Here's how the part is built. I have some questions about the finished solid (model axes, mm). A direction names the side the tool comes from. Round coordinates to 2 decimals unless told otherwise and drop trailing zeros. Order: outer loops, then holes, each group sorted by start corner. A loop starts at its lowest first (then second) coordinate and runs counter-clockwise, first axis right, second up. Notation, with made-up numbers: M 80,-39 L 120,-39 A28 cw 120,-18 Z; hole C -13.75,73.5 d6. An arc over 180 degrees is marked long. Write each question's results on one line, items separated by ' | '. Start each with the question number.
```python
from build123d import *

# Parameters (mm, degrees)
SKETCH1_W           = 15.000000596
SKETCH1_H           = 15.000000597
BOSS_EXTRUDE1_DEPTH = 12.000000104
SKETCH2_W           = 8.999999613
SKETCH2_H           = 9.000003338
CUT_EXTRUDE1_DEPTH  = 11.002000072
SKETCH3_W           = 6.504997611
SKETCH3_H           = 6.504997611
CUT_EXTRUDE2_DEPTH  = 102.11874099
SKETCH4_W           = 3.00199911
SKETCH4_H           = 7.001999765
CUT_EXTRUDE3_DEPTH  = 1.501999795
SKETCH5_W           = 7.001999765
SKETCH5_H           = 3.002002835
CUT_EXTRUDE4_DEPTH  = 1.501999795
SKETCH6_W           = 7.001999765
SKETCH6_H           = 3.002002835
CUT_EXTRUDE5_DEPTH  = 1.502998173
SKETCH7_W           = 3.00199911
SKETCH7_H           = 7.001999765
CUT_EXTRUDE6_DEPTH  = 1.502998173
SKETCH9_W           = 2
SKETCH9_H           = 5.000000597
BOSS_EXTRUDE2_DEPTH = 5
SKETCH10_W          = 2
SKETCH10_H          = 5.000000597
BOSS_EXTRUDE3_DEPTH = 5
SKETCH11_R          = 1.6
CUT_EXTRUDE7_DEPTH  = 5


with BuildPart() as part:
    # Sketch1 → Boss-Extrude1 (new body)
    with BuildSketch(Plane(origin=(0, 0, 0), x_dir=(-1, 0, 0), z_dir=(0, 0, -1))):
        with Locations((47.499999404, 76.49999857)):
            Rectangle(SKETCH1_W, SKETCH1_H)
    extrude(amount=-BOSS_EXTRUDE1_DEPTH)

    # Sketch2 → Cut-Extrude1 (cut)
    with BuildSketch(Plane.XY.offset(12.000000104)):
        with Locations((-47.500001266, 76.375000179)):
            Rectangle(SKETCH2_W, SKETCH2_H)
    extrude(amount=-CUT_EXTRUDE1_DEPTH, mode=Mode.SUBTRACT)

    # Sketch3 → Cut-Extrude2 (cut, through all)
    with BuildSketch(Plane(origin=(0, 0, 0), x_dir=(-1, 0, 0), z_dir=(0, 0, -1))):
        with Locations((47.500498593, 76.375499367)):
            Rectangle(SKETCH3_W, SKETCH3_H)
    extrude(amount=-CUT_EXTRUDE2_DEPTH, mode=Mode.SUBTRACT)

    # Sketch4 → Cut-Extrude3 (cut)
    with BuildSketch(Plane(origin=(0, 71.87499851, 0), x_dir=(-1, 0, 0), z_dir=(0, 1, 0))):
        with Locations((47.500001267, 8.499000222)):
            Rectangle(SKETCH4_W, SKETCH4_H)
    extrude(amount=-CUT_EXTRUDE3_DEPTH, mode=Mode.SUBTRACT)

    # Sketch5 → Cut-Extrude4 (cut)
    with BuildSketch(Plane.ZY.offset(43.00000146)):
        with Locations((8.499000222, 76.375000179)):
            Rectangle(SKETCH5_W, SKETCH5_H)
    extrude(amount=-CUT_EXTRUDE4_DEPTH, mode=Mode.SUBTRACT)

    # Sketch6 → Cut-Extrude5 (cut)
    with BuildSketch(Plane(origin=(-52.000001073, 0, 0), x_dir=(0, 0, -1), z_dir=(1, 0, 0))):
        with Locations((-8.499000222, 76.375000179)):
            Rectangle(SKETCH6_W, SKETCH6_H)
    extrude(amount=-CUT_EXTRUDE5_DEPTH, mode=Mode.SUBTRACT)

    # Sketch7 → Cut-Extrude6 (cut)
    with BuildSketch(Plane.XZ.offset(-80.875001848)):
        with Locations((-47.500001267, 8.499000222)):
            Rectangle(SKETCH7_W, SKETCH7_H)
    extrude(amount=-CUT_EXTRUDE6_DEPTH, mode=Mode.SUBTRACT)

    # Sketch9 → Boss-Extrude2 (add)
    with BuildSketch(Plane.ZY.offset(54.999999702)):
        with Locations((1, 76.49999857)):
            Rectangle(SKETCH9_W, SKETCH9_H)
    extrude(amount=BOSS_EXTRUDE2_DEPTH)

    # Sketch10 → Boss-Extrude3 (add)
    with BuildSketch(Plane(origin=(-39.999999106, 0, 0), x_dir=(0, 0, -1), z_dir=(1, 0, 0))):
        with Locations((-1, 76.49999857)):
            Rectangle(SKETCH10_W, SKETCH10_H)
    extrude(amount=BOSS_EXTRUDE3_DEPTH)

    # Sketch11 → Cut-Extrude7 (cut)
    with BuildSketch(Plane.XY.offset(2)):
        with Locations((-37.499999106, 76.499998569)):
            Circle(SKETCH11_R)
        with Locations((-57.499999702, 76.499998569)):
            Circle(SKETCH11_R)
    extrude(amount=-CUT_EXTRUDE7_DEPTH, mode=Mode.SUBTRACT)


solid = part.part
```
(1) I want a section at B-B on z = 7.75. Write out the boundary of the cut face in (x, y) (3 decimals).
(2) I want a section at A-A on x = -37.5. Write out the boundary of the cut face in (y, z), and give its area (3 significant figures).
(3) If we mould it in two halves opening along Y, with no side actions, what happens to faces 4 (the flat face through (-47, 80, 0)), 5 (the flat face through (-48, 82.378, 9)), 6 (the flat face through (-38, 79, 1))? For each: pulls with the +Y half, pulls with the -Y half, needs draft (parallel to the pull), parting line crosses it, or undercut.
(4) Please list where these lines run through material, in increasing order: line 1 (Y direction, x = -57.5, z = 1.3); line 2 (Y direction, x = -44.5, z = 10.25) (3 decimals); line 3 (X direction, y = 78.75, z = 6.75).
(5) I want a section at D-D on x = -45.5. Write out the boundary of the cut face in (y, z) (3 decimals), and give its area (3 significant figures).
(6) I'm going to push flat-ended pins straight in: pin 1 Ø4.5 at (x, y) = (-49, 77) entering from +Z; pin 2 Ø1.5 at (y, z) = (75.5, 5) entering from -X; pin 3 Ø1.2 at (y, z) = (71, 8) entering from +X. Where does each tip first touch, or does it pass through?
(7) I want a section at C-C on y = 72.75. Write out the boundary of the cut face in (x, z), and give its area (3 significant figures).
(8) On a 3-axis mill with a long thin cutter (end or side, diameter ignored), from which of +Z, -Z, +X, -X, +Y, -Y can I reach the whole of each face in a straight line? I mean faces 1 (the flat face through (-42, 77.876, 8)), 2 (the flat face through (-56, 75, 2)), 3 (the flat face through (-39, 75, 2)). Say none if no direction works.
Solutions:
1) outline: M -55,69 L -40,69 L -40,84 L -55,84 Z; hole M -53.503,74.874 L -52,74.874 L -52,71.875 L -49.001,71.875 L -49.001,70.373 L -45.999,70.373 L -45.999,71.875 L -43,71.875 L -43,74.874 L -41.498,74.874 L -41.498,77.876 L -43,77.876 L -43,80.875 L -45.999,80.875 L -45.999,82.378 L -49.001,82.378 L -49.001,80.875 L -52,80.875 L -52,77.876 L -53.503,77.876 Z
2) outline: M 74,0 L 74.9,0 L 74.9,2 L 74,2 Z; M 78.1,0 L 79,0 L 79,2 L 78.1,2 Z | area: 3.60 mm^2
3) face 4: needs draft | face 5: undercut | face 6: pulls with the +Y half
4) line 1: 74 to 74.9, 78.1 to 79 | line 2: 69 to 71.875, 80.875 to 84 | line 3: -55 to -52, -43 to -40
5) outline: M 69,0 L 73.123,0 L 73.123,0.998 L 71.875,0.998 L 71.875,12 L 69,12 Z; M 79.628,0 L 84,0 L 84,12 L 80.875,12 L 80.875,0.998 L 79.628,0.998 Z | area: 74.5 mm^2
6) pin 1: z = 1 | pin 2: x = -55 | pin 3: x = -40
7) outline: M -55,0 L -40,0 L -40,12 L -43,12 L -43,1 L -52,1 L -52,12 L -55,12 Z | area: 81.0 mm^2
8) face 1: +Z | face 2: +Z, -X, +Y, -Y | face 3: +Z, +X, +Y, -Y
